```python
from build123d import *

# Parameters (mm, degrees)
SKETCH1_R           = 4
SKETCH1_R_2         = 1.6
BOSS_EXTRUDE1_DEPTH = 5.4
BOSS_EXTRUDE2_START = -2.1
SKETCH2_R           = 1.6
SKETCH2_R_2         = 0.65
BOSS_EXTRUDE2_DEPTH = 2.1
SKETCH3_R           = 2.5
CUT_EXTRUDE1_DEPTH  = 3.7


with BuildPart() as part:
    # Sketch1 → Boss-Extrude1 (new body)
    with BuildSketch(Plane.XY):
        with Locations(Location((0, 0, 0), (0, 0, 180))):
            Circle(SKETCH1_R)
        with Locations(Location((0, 0, 0), (0, 0, 180))):
            Circle(SKETCH1_R_2, mode=Mode.SUBTRACT)
    extrude(amount=BOSS_EXTRUDE1_DEPTH)

    # Sketch2 → Boss-Extrude2 (add)
    with BuildSketch(Plane.XY.offset(5.4).offset(BOSS_EXTRUDE2_START)):
        with BuildLine():
            Line((4.171930009, 4.171930009), (3.333452378, 5.01040764))
            ThreePointArc((3.333452378, 5.01040764), (3.116679627, 5.334830989), (3.040559159, 5.717514421))
            Line((3.040559159, 5.717514421), (3.040559159, 7.94985144))
            ThreePointArc((3.040559159, 7.94985144), (3.039133792, 8.003224674), (3.034861755, 8.056445754))
            Line((3.034861755, 8.056445754), (1.99577765, 17.748932949))
            ThreePointArc((1.99577765, 17.748932949), (1.669833374, 18.386178105), (1.001475054, 18.642338635))
            Line((1.001475054, 18.642338635), (-1.001475054, 18.642338635))
            ThreePointArc((-1.001475054, 18.642338635), (-1.669833374, 18.386178105), (-1.99577765, 17.748932949))
            Line((-1.99577765, 17.748932949), (-3.034861755, 8.056445754))
            ThreePointArc((-3.034861755, 8.056445754), (-3.039133792, 8.003224674), (-3.040559159, 7.94985144))
            Line((-3.040559159, 7.94985144), (-3.040559159, 5.717514421))
            ThreePointArc((-3.040559159, 5.717514421), (-3.116679627, 5.334830989), (-3.333452378, 5.01040764))
            Line((-3.333452378, 5.01040764), (-4.171930009, 4.171930009))
            Line((-4.171930009, 4.171930009), (-5.01040764, 3.333452378))
            ThreePointArc((-5.01040764, 3.333452378), (-5.334830989, 3.116679627), (-5.717514421, 3.040559159))
            Line((-5.717514421, 3.040559159), (-7.94985144, 3.040559159))
            ThreePointArc((-7.94985144, 3.040559159), (-8.003224674, 3.039133792), (-8.056445754, 3.034861755))
            Line((-8.056445754, 3.034861755), (-17.748932949, 1.99577765))
            ThreePointArc((-17.748932949, 1.99577765), (-18.386178105, 1.669833374), (-18.642338635, 1.001475054))
            Line((-18.642338635, 1.001475054), (-18.642338635, -1.001475054))
            ThreePointArc((-18.642338635, -1.001475054), (-18.386178105, -1.669833374), (-17.748932949, -1.99577765))
            Line((-17.748932949, -1.99577765), (-8.056445754, -3.034861755))
            ThreePointArc((-8.056445754, -3.034861755), (-8.003224674, -3.039133792), (-7.94985144, -3.040559159))
            Line((-7.94985144, -3.040559159), (-5.717514421, -3.040559159))
            ThreePointArc((-5.717514421, -3.040559159), (-5.334830989, -3.116679627), (-5.01040764, -3.333452378))
            Line((-5.01040764, -3.333452378), (-4.171930009, -4.171930009))
            Line((-4.171930009, -4.171930009), (-3.333452378, -5.01040764))
            ThreePointArc((-3.333452378, -5.01040764), (-3.116679627, -5.334830989), (-3.040559159, -5.717514421))
            Line((-3.040559159, -5.717514421), (-3.040559159, -7.94985144))
            ThreePointArc((-3.040559159, -7.94985144), (-3.039133792, -8.003224674), (-3.034861755, -8.056445754))
            Line((-3.034861755, -8.056445754), (-1.99577765, -17.748932949))
            ThreePointArc((-1.99577765, -17.748932949), (-1.669833374, -18.386178105), (-1.001475054, -18.642338635))
            Line((-1.001475054, -18.642338635), (1.001475054, -18.642338635))
            ThreePointArc((1.001475054, -18.642338635), (1.669833374, -18.386178105), (1.99577765, -17.748932949))
            Line((1.99577765, -17.748932949), (3.034861755, -8.056445754))
            ThreePointArc((3.034861755, -8.056445754), (3.039133792, -8.003224674), (3.040559159, -7.94985144))
            Line((3.040559159, -7.94985144), (3.040559159, -5.717514421))
            ThreePointArc((3.040559159, -5.717514421), (3.116679627, -5.334830989), (3.333452378, -5.01040764))
            Line((3.333452378, -5.01040764), (4.171930009, -4.171930009))
            Line((4.171930009, -4.171930009), (5.01040764, -3.333452378))
            ThreePointArc((5.01040764, -3.333452378), (5.334830989, -3.116679627), (5.717514421, -3.040559159))
            Line((5.717514421, -3.040559159), (7.94985144, -3.040559159))
            ThreePointArc((7.94985144, -3.040559159), (8.003224674, -3.039133792), (8.056445754, -3.034861755))
            Line((8.056445754, -3.034861755), (17.748932949, -1.99577765))
            ThreePointArc((17.748932949, -1.99577765), (18.386178105, -1.669833374), (18.642338635, -1.001475054))
            Line((18.642338635, -1.001475054), (18.642338635, 1.001475054))
            ThreePointArc((18.642338635, 1.001475054), (18.386178105, 1.669833374), (17.748932949, 1.99577765))
            Line((17.748932949, 1.99577765), (8.056445754, 3.034861755))
            ThreePointArc((8.056445754, 3.034861755), (8.003224674, 3.039133792), (7.94985144, 3.040559159))
            Line((7.94985144, 3.040559159), (5.717514421, 3.040559159))
            ThreePointArc((5.717514421, 3.040559159), (5.334830989, 3.116679627), (5.01040764, 3.333452378))
            Line((5.01040764, 3.333452378), (4.171930009, 4.171930009))
        make_face()
        with Locations(Location((0, 0, 0), (0, 0, 180))):
            Circle(SKETCH2_R, mode=Mode.SUBTRACT)
        with Locations((0, 6.1)):
            Circle(SKETCH2_R_2, mode=Mode.SUBTRACT)
        with Locations((0, 9.3)):
            Circle(SKETCH2_R_2, mode=Mode.SUBTRACT)
        with Locations((0, 12.5)):
            Circle(SKETCH2_R_2, mode=Mode.SUBTRACT)
        with Locations((0, 15.7)):
            Circle(SKETCH2_R_2, mode=Mode.SUBTRACT)
        with Locations((15.7, 0)):
            Circle(SKETCH2_R_2, mode=Mode.SUBTRACT)
        with Locations((12.5, 0)):
            Circle(SKETCH2_R_2, mode=Mode.SUBTRACT)
        with Locations((9.3, 0)):
            Circle(SKETCH2_R_2, mode=Mode.SUBTRACT)
        with Locations((6.1, 0)):
            Circle(SKETCH2_R_2, mode=Mode.SUBTRACT)
        with Locations((0, -15.7)):
            Circle(SKETCH2_R_2, mode=Mode.SUBTRACT)
        with Locations((0, -12.5)):
            Circle(SKETCH2_R_2, mode=Mode.SUBTRACT)
        with Locations((0, -9.3)):
            Circle(SKETCH2_R_2, mode=Mode.SUBTRACT)
        with Locations((0, -6.1)):
            Circle(SKETCH2_R_2, mode=Mode.SUBTRACT)
        with Locations((-15.7, 0)):
            Circle(SKETCH2_R_2, mode=Mode.SUBTRACT)
        with Locations((-12.5, 0)):
            Circle(SKETCH2_R_2, mode=Mode.SUBTRACT)
        with Locations((-9.3, 0)):
            Circle(SKETCH2_R_2, mode=Mode.SUBTRACT)
        with Locations((-6.1, 0)):
            Circle(SKETCH2_R_2, mode=Mode.SUBTRACT)
    extrude(amount=BOSS_EXTRUDE2_DEPTH)

    # Sketch3 → Cut-Extrude1 (cut)
    with BuildSketch(Plane(origin=(0, 0, 0), x_dir=(-1, 0, 0), z_dir=(0, 0, -1))):
        Circle(SKETCH3_R)
    extrude(amount=-CUT_EXTRUDE1_DEPTH, mode=Mode.SUBTRACT)


solid = part.part
```
Work out the finished part from the listing and answer in its coordinate system (mm). A direction names the side the tool comes from. Give positions to 0.01 mm unless a question says otherwise; leave off trailing zeros. Loops run counter-clockwise (first coordinate to the right, second up) from the corner with the lowest first, then second, coordinate; pieces in that order, holes last. Notation, with made-up numbers: M 18.25,79.25 L 30.25,79.25 A27 cw 30.25,113.25 Z; hole C -24.75,86.25 d8. An arc over 180 degrees is marked long. One line per item, written item: value. Start each with the question number.
1. Each of these flat-tipped pins is pushed along its axis until it touches: P1, Ø1.7, axis at x = 0, y = -9.3, coming from the -Z side; P2, Ø1, axis at y = -6.5, z = 4, coming from the +X side; P3, Ø1, axis at x = -9.3, y = 0, coming from the -Z side; P4, Ø2.5, axis at y = -6.5, z = 4.5, coming from the -X side. Where does it stop, or does it pass through?
2. Which of the six approach directions +Z, -Z, +X, -X, +Y, -Y give full straight-line access (tool end or side, diameter ignored) to faces 1 (the face through (0.867, 3.905, 1.627)), 2 (the face through (-7, 3.041, 4)), 3 (the face through (3.041, -7, 4))?
3. Find section A-A (y = -12.5). Give the vertices of the cut face in (x, z).
4. Find section D-D (z = 1.4). Give the vertices of the cut face in (x, y).
5. Find the intervals of material crossed by probe 1 along X at (y, z) = (6, 4.1); probe 2 along Y at (x, z) = (-6.1, 3.95); probe 3 along Z at (x, y) = (13, -2), in increasing order.
6. Determine the mould class of faces 4 (the face through (-1.526, -0.481, 4.538)), 5 (the face through (5.45, 0.03, 4.34)), 6 (the face through (-4.184, -4.16, 4.335)), 7 (the face through (1.677, 18.379, 4.335)) for opening direction Y: released by +Y, released by -Y, zero draft, split by the parting line, or undercut.
7. Find section C-C (z = 4.85). State how many separate pieces and enclosed holes the cut face has, and give its area (3 significant figures).
Reported:
1. P1: stops at z = 3.3
1. P2: stops at x = 3.04
1. P3: passes through
1. P4: stops at x = -3.16
2. face 1: -Z
2. face 2: +Z, -Z, -X, +Y
2. face 3: +Z, -Z, +X, -Y
3. outline: M -2.56,3.3 L -0.65,3.3 L -0.65,5.4 L -2.56,5.4 Z; M 0.65,3.3 L 2.56,3.3 L 2.56,5.4 L 0.65,5.4 Z
4. outline: C 0,0 d8; hole C 0,0 d5
5. probe 1: x = -3.04 to -0.64, 0.64 to 3.04
5. probe 2: y = -3.04 to -0.65, 0.65 to 3.04
5. probe 3: z = 3.3 to 5.4
6. face 4: undercut
6. face 5: undercut
6. face 6: released by -Y
6. face 7: released by +Y
7. separate pieces: 1
7. enclosed holes: 17
7. area: 348 mm²
